Geometry: final body of the model. Coordinates: model frame, mm. Coordinates: 2 decimals unless noted, no trailing zeros. Order: outer loops, then holes, each group sorted by start corner. A loop starts at its lowest first (then second) coordinate and runs counter-clockwise, first axis right, second up. Notation, with made-up numbers: M 61.5,-17.75 L 106.5,-17.75 A23 ccw 106.5,-0.75 Z; hole C 11,44.25 d3. An arc over 180 degrees is marked long. Write item = value, one per line.
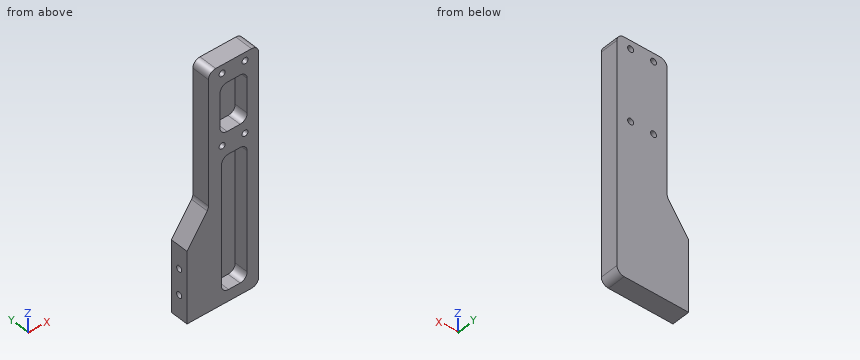
from build123d import *

# Parameters (mm, degrees)
SKETCH12_W                = 50
SKETCH12_H                = 12.7
BOSS_EXTRUDE1_DEPTH       = 112
M5X0_8_TAPPED_HOLE3_D     = 4.2
SKETCH19_W                = 50
SKETCH19_H                = 12.7
BOSS_EXTRUDE2_DEPTH       = 53
M5X0_8_TAPPED_HOLE4_D     = 4.2
M5X0_8_TAPPED_HOLE4_DEPTH = 20
M5X0_8_TAPPED_HOLE4_TIP   = 1.2618073
CUT_EXTRUDE1_DEPTH        = 116.456875066
SKETCH26_3_W              = 19
SKETCH26_3_H              = 33.9
SKETCH26_3_W_2            = 18
SKETCH26_3_H_2            = 93.3
CUT_EXTRUDE2_DEPTH        = 9.7
FILLET1_R                 = 5


with BuildPart() as part:
    # Sketch12 → Boss-Extrude1 (new body)
    with BuildSketch(Plane.XY):
        Rectangle(SKETCH12_W, SKETCH12_H)
    extrude(amount=BOSS_EXTRUDE1_DEPTH)

    # M5x0.8 Tapped Hole3 (through all)
    with Locations(Plane(origin=(0, 6.35, 0), x_dir=(1, 0, 0), z_dir=(0, 1, 0))):
        with Locations((-0.5, -56.3), (15.5, -56.3), (15.5, -106.2), (-0.5, -106.2)):
            Hole(M5X0_8_TAPPED_HOLE3_D / 2)

    # Sketch19 → Boss-Extrude2 (add)
    with BuildSketch(Plane(origin=(0, 0, 0), x_dir=(-1, 0, 0), z_dir=(0, 0, -1))):
        Rectangle(SKETCH19_W, SKETCH19_H)
    extrude(amount=BOSS_EXTRUDE2_DEPTH)

    # M5x0.8 Tapped Hole4
    with Locations(Plane.ZY.offset(25)):
        with Locations((-37, 0), (-19, 0)):
            Hole(M5X0_8_TAPPED_HOLE4_D / 2, depth=M5X0_8_TAPPED_HOLE4_DEPTH)
            with Locations((0, 0, -(M5X0_8_TAPPED_HOLE4_DEPTH + M5X0_8_TAPPED_HOLE4_TIP / 2))):  # 118° drill point
                Cone(0, M5X0_8_TAPPED_HOLE4_D / 2, M5X0_8_TAPPED_HOLE4_TIP, mode=Mode.SUBTRACT)

    # Sketch26 → Cut-Extrude1 (cut, through all)
    with BuildSketch(Plane.XZ.offset(6.35)):
        Polygon((-10, 18.422220101), (-10, 112), (-25, 112), (-25, -3), align=None)
    extrude(amount=-CUT_EXTRUDE1_DEPTH, mode=Mode.SUBTRACT)

    # Sketch26_3 → Cut-Extrude2 (cut)
    with BuildSketch(Plane.XZ.offset(6.35)):
        with Locations((7.5, 81.25)):
            Rectangle(SKETCH26_3_W, SKETCH26_3_H)
        with Locations((8, 1.65)):
            Rectangle(SKETCH26_3_W_2, SKETCH26_3_H_2)
    extrude(amount=-CUT_EXTRUDE2_DEPTH, mode=Mode.SUBTRACT)

    # Fillet1
    fillet1_edges = [part.edges().sort_by_distance(p)[0] for p in [
        (25, 0, -53),
        (25, 0, 112),
        (-10, 0, 18.422220101),
        (-10, 0, 112),
        (-2, -1.5, 98.2),
        (17, -1.5, 98.2),
        (17, -1.5, 64.3),
        (-2, -1.5, 64.3),
        (-1, -1.5, -45),
        (-1, -1.5, 48.3),
        (17, -1.5, 48.3),
        (17, -1.5, -45),
    ]]
    fillet(fillet1_edges, radius=FILLET1_R)


solid = part.part
1) Section B-B, the plane x = 15.5. Return loops of the section in (y, z).
Numbers:
outline = M -6.35,-53 L 6.35,-53 L 6.35,54.2 L -6.35,54.2 L -6.35,46.87 L 3.35,46.87 L 3.35,-43.57 L -6.35,-43.57 Z; M -6.35,58.4 L 6.35,58.4 L 6.35,104.1 L -6.35,104.1 L -6.35,96.77 L 3.35,96.77 L 3.35,65.73 L -6.35,65.73 Z; M -6.35,108.3 L 6.35,108.3 L 6.35,112 L -6.35,112 Z
2) Section D-D, the plane x = -21. Return loops of the section in (y, z).
Numbers:
outline = M -6.35,-53 L 6.35,-53 L 6.35,2.71 L -6.35,2.71 Z; hole C 0,-37 d4.2; hole C 0,-19 d4.2
3) Pin query (flat end, axial travel): pin 1 (5 mm diameter, centred on y = -0.5, z = 81.5, fed in from -X). Return the tip coordinate at first contact, or that it passes through.
Numbers:
pin_1 = -10
4) Line query: L1, parallel to X at y = 2.25, z = 56.3; L2, parallel to Z at x = -21, y = -1.5; L3, parallel to X at y = 0.75, z = -31. Output: solid intervals per line, ascending.
Numbers:
L1 = -10 to -2.6, 1.6 to 13.4, 17.6 to 25
L2 = -53 to -38.47, -35.53 to -20.47, -17.53 to 2.71
L3 = -25 to -1, 17 to 25
5) Section A-A, the plane z = 56.3. Return loops of the section in (x, y).
Numbers:
outline = M -10,-6.35 L -2.6,-6.35 L -2.6,6.35 L -10,6.35 Z; M 1.6,-6.35 L 13.4,-6.35 L 13.4,6.35 L 1.6,6.35 Z; M 17.6,-6.35 L 25,-6.35 L 25,6.35 L 17.6,6.35 Z
6) Section C-C, the plane z = 4. Return loops of the section in (x, y), and give its area (3 significant figures).
Numbers:
outline = M -20.1,-6.35 L -1,-6.35 L -1,3.35 L 17,3.35 L 17,-6.35 L 25,-6.35 L 25,6.35 L -20.1,6.35 Z
area = 398 mm²
